```python
from build123d import *

# Parameters (mm, degrees)
EXTRUDE_1_DEPTH     = 4
SKETCH_3_R          = 18.5
CUT_EXTRUDE_2_DEPTH = 256.679975751
SKETCH_6_R          = 2.1
CUT_EXTRUDE_5_DEPTH = 256.679975751
SKETCH_7_W          = 25
SKETCH_7_H          = 65
CUT_EXTRUDE_6_DEPTH = 256.679975751
SKETCH_8_R          = 1
CUT_EXTRUDE_7_DEPTH = 256.679975751
SKETCH_9_R          = 1.6
CUT_EXTRUDE_8_DEPTH = 256.679975751
SKETCH_10_W         = 50
SKETCH_10_H         = 20
CUT_EXTRUDE_9_DEPTH = 256.679975751
FILLET_2_R          = 5


with BuildPart() as part:
    # 草图1 → 凸台-拉伸1 (new body)
    with BuildSketch(Plane.XY):
        with BuildLine():
            Line((-212.5, 40), (212.5, 40))
            ThreePointArc((212.5, 40), (252.5, 0), (212.5, -40))
            Line((212.5, -40), (-212.5, -40))
            ThreePointArc((-212.5, -40), (-252.5, 0), (-212.5, 40))
        make_face()
    extrude(amount=EXTRUDE_1_DEPTH)

    # 草图3 → 切除-拉伸2 (cut, through all)
    with BuildSketch(Plane.XY.offset(4)):
        with Locations((-212.5, 0)):
            Circle(SKETCH_3_R)
        with Locations((212.5, 0)):
            Circle(SKETCH_3_R)
    extrude(amount=-CUT_EXTRUDE_2_DEPTH, mode=Mode.SUBTRACT)

    # 草图6 → 切除-拉伸5 (cut, through all)
    with BuildSketch(Plane(origin=(0, 0, 0), x_dir=(-1, 0, 0), z_dir=(0, 0, -1))):
        with Locations((-247.5, 0)):
            Circle(SKETCH_6_R)
        with Locations((-237.248737342, 24.748737342)):
            Circle(SKETCH_6_R)
        with Locations((-212.5, 35)):
            Circle(SKETCH_6_R)
        with Locations((-187.751262658, 24.748737342)):
            Circle(SKETCH_6_R)
        with Locations((-177.5, 0)):
            Circle(SKETCH_6_R)
        with Locations((-187.751262658, -24.748737342)):
            Circle(SKETCH_6_R)
        with Locations((-212.5, -35)):
            Circle(SKETCH_6_R)
        with Locations((-237.248737342, -24.748737342)):
            Circle(SKETCH_6_R)
    cut_extrude_5 = extrude(amount=-CUT_EXTRUDE_5_DEPTH, mode=Mode.SUBTRACT)

    # 镜向1: 切除-拉伸5 across plane
    add(cut_extrude_5.mirror(Plane(origin=(0, 0, 0), x_dir=(0, 0, 1), z_dir=(1, 0, 0))), mode=Mode.SUBTRACT)

    # 草图7 → 切除-拉伸6 (cut, through all)
    with BuildSketch(Plane(origin=(0, 0, 0), x_dir=(-1, 0, 0), z_dir=(0, 0, -1))):
        Rectangle(SKETCH_7_W, SKETCH_7_H)
    extrude(amount=-CUT_EXTRUDE_6_DEPTH, mode=Mode.SUBTRACT)

    # 草图8 → 切除-拉伸7 (cut, through all)
    with BuildSketch(Plane(origin=(0, 0, 0), x_dir=(-1, 0, 0), z_dir=(0, 0, -1))):
        with Locations((-12.5, 32.5)):
            Circle(SKETCH_8_R)
        with Locations((12.5, 32.5)):
            Circle(SKETCH_8_R)
        with Locations((-12.5, -32.5)):
            Circle(SKETCH_8_R)
        with Locations((12.5, -32.5)):
            Circle(SKETCH_8_R)
    extrude(amount=-CUT_EXTRUDE_7_DEPTH, mode=Mode.SUBTRACT)

    # 草图9 → 切除-拉伸8 (cut, through all)
    with BuildSketch(Plane(origin=(0, 0, 0), x_dir=(-1, 0, 0), z_dir=(0, 0, -1))):
        with Locations((-15.5, -4.5)):
            Circle(SKETCH_9_R)
        with Locations(Location((-15.5, 4.5, 0), (0, 0, 180))):
            Circle(SKETCH_9_R)
        with Locations(Location((15.5, -4.5, 0), (0, 0, 180))):
            Circle(SKETCH_9_R)
        with Locations((15.5, 4.5)):
            Circle(SKETCH_9_R)
    extrude(amount=-CUT_EXTRUDE_8_DEPTH, mode=Mode.SUBTRACT)

    # 草图10 → 切除-拉伸9 (cut, through all)
    with BuildSketch(Plane.XY.offset(4)):
        with Locations((100, -24)):
            Rectangle(SKETCH_10_W, SKETCH_10_H)
        with Locations((-100, 24)):
            Rectangle(SKETCH_10_W, SKETCH_10_H)
    extrude(amount=-CUT_EXTRUDE_9_DEPTH, mode=Mode.SUBTRACT)

    # 圆角2
    fillet_2_edges = [part.edges().sort_by_distance(p)[0] for p in [
        (75, -34, 2),
        (75, -14, 2),
        (125, -14, 2),
        (125, -34, 2),
        (-125, 34, 2),
        (-75, 34, 2),
        (-75, 14, 2),
        (-125, 14, 2),
    ]]
    fillet(fillet_2_edges, radius=FILLET_2_R)


solid = part.part
```
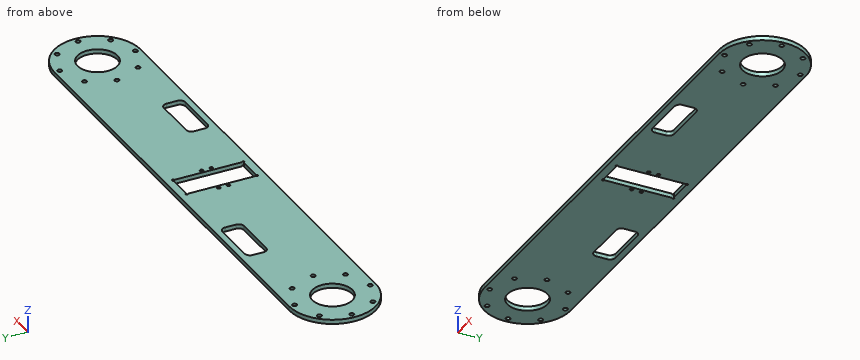
Input: part model. Units: mm. Frame: model coordinates. Coordinates: 2 decimals unless noted, no trailing zeros. Loops run counter-clockwise (first coordinate to the right, second up) from the corner with the lowest first, then second, coordinate; pieces in that order, holes last. Notation, with made-up numbers: (33.25, 81) - (88.25, 81) arc R19 ccw to (88.25, 90) - close; hole circle Ø5 at (71, 56). An arc over 180 degrees is marked (long way). Answer in a Markdown table with one row per item.
(1) Material intervals for L1, parallel to X at y = 20.5, z = 1.15; L2, parallel to Y at x = -14.5, z = 2.2; L3, parallel to X at y = -28.5, z = 2.15, sorted ascending. Write a range as from..to.
Model answer:
| item | result |
|---|---|
| L1 | x = -246.85..-125, -75..-12.5, 12.5..246.85 |
| L2 | y = -40..-5.75, -3.25..3.25, 5.75..40 |
| L3 | x = -240.57..-12.5, 12.5..75, 125..240.57 |
(2) Cut plane C-C on z = 2.6. Count the separate pieces of the cut face and the enclosed holes in it, plus the area to 3 significant figures.
Model answer:
| item | result |
|---|---|
| separate pieces | 1 |
| enclosed holes | 25 |
| area | 33,000 mm² |
(3) Cut plane B-B on x = -200. Output: boundary loops of the cut face in (y, z), plus the area to 3 significant figures.
Model answer:
| item | result |
|---|---|
| outline | (-40, 0) - (-13.64, 0) - (-13.64, 4) - (-40, 4) - close; (13.64, 0) - (40, 0) - (40, 4) - (13.64, 4) - close |
| area | 211 mm² |
(4) Cut plane A-A on x = -91. Output: boundary loops of the cut face in (y, z), plus the area to 3 significant figures.
Model answer:
| item | result |
|---|---|
| outline | (-40, 0) - (14, 0) - (14, 4) - (-40, 4) - close; (34, 0) - (40, 0) - (40, 4) - (34, 4) - close |
| area | 240 mm² |
